Can you work these out from the model? Positions are in its coordinate system, mm. Coordinates: 2 decimals unless noted, no trailing zeros. Order: outer loops, then holes, each group sorted by start corner. A loop starts at its lowest first (then second) coordinate and runs counter-clockwise, first axis right, second up. Notation, with made-up numbers: (71.5, -12) -> (92.5, -12) arc R20 ccw to (92.5, 7) -> close; hole circle Ø7 at (39.5, -17.5). An arc over 180 degrees is marked (long way). Return JSON: item names as keys, results as strings. Group by question number.
1) If we section it at D-D, the plane z = -8: Please give me the cut outline in (x, y).
2) If I drill on probe 1 along Z at (x, y) = (0, 38.6) (3 decimals); probe 2 along Y at (x, z) = (2.25, 0) (3 decimals); probe 3 along Y at (x, z) = (0, -7), over which ranges is the centre line in solid material (lowest first)? Write a range as from..to.
3) If we section it at C-C, the plane x = 0.75: Please give me the cut outline in (y, z) (3 decimals).
4) Thinking about a two-plate mould opening in X: for faces 1 (the flat face through (4, 16, 16)), 2 (the flat face through (-2, 0, 0)), 3 (the cylindrical face through (-0.2, 20.95, -20.86)), 4 (the flat face through (-4, 16, 16)), which applies, +X half, -X half, draft (parallel to the pull), parting line (faces both ways), or undercut?
5) If we section it at A-A, the plane y = 25.5: Please give me the cut outline in (x, z) (1 decimal).
6) If we section it at B-B, the plane z = 0: Please give me the cut outline in (x, y) (1 decimal).
from build123d import *

# Parameters (mm, degrees)
SKETCH2_W           = 8.001
SKETCH2_H           = 45.75
SKETCH2_R           = 1.5
BOSS_EXTRUDE1_DEPTH = 42.5
SKETCH3_R           = 15.875
CUT_EXTRUDE1_DEPTH  = 42.5


with BuildPart() as part:
    # Sketch2 → Boss-Extrude1 (new body)
    with BuildSketch(Plane(origin=(0, 0, 0), x_dir=(1, 0, 0), z_dir=(0, 1, 0))):
        Rectangle(SKETCH2_W, SKETCH2_H)
        Circle(SKETCH2_R, mode=Mode.SUBTRACT)
        with Locations((0, 19.375)):
            Circle(SKETCH2_R, mode=Mode.SUBTRACT)
        with Locations((0, -19.375)):
            Circle(SKETCH2_R, mode=Mode.SUBTRACT)
    extrude(amount=BOSS_EXTRUDE1_DEPTH)

    # Sketch3 → Cut-Extrude1 (cut)
    with BuildSketch(Plane(origin=(4.0005, 0, 0), x_dir=(0, 0, -1), z_dir=(1, 0, 0))):
        with Locations((0, 21.25)):
            Circle(SKETCH3_R)
    extrude(amount=-CUT_EXTRUDE1_DEPTH, mode=Mode.SUBTRACT)


solid = part.part
Result sheet:
{
 "1": {"outline": "(-4, 0) -> (4, 0) -> (4, 7.54) -> (-4, 7.54) -> close; (-4, 34.96) -> (4, 34.96) -> (4, 42.5) -> (-4, 42.5) -> close"},
 "2": {"probe 1": "z = -22.875..-20.875, -17.875..-1.5, 1.5..17.875, 20.875..22.875", "probe 2": "y = 0..5.375, 37.125..42.5", "probe 3": "y = 0..7, 35.5..42.5"},
 "3": {"outline": "(0, -22.875) -> (42.5, -22.875) -> (42.5, -20.674) -> (0, -20.674) -> close; (0, -18.076) -> (42.5, -18.076) -> (42.5, -1.299) -> (37.072, -1.299) arc R15.875 cw to (5.428, -1.299) -> (0, -1.299) -> close; (0, 1.299) -> (5.428, 1.299) arc R15.875 cw to (37.072, 1.299) -> (42.5, 1.299) -> (42.5, 18.076) -> (0, 18.076) -> close; (0, 20.674) -> (42.5, 20.674) -> (42.5, 22.875) -> (0, 22.875) -> close"},
 "4": {"face 1": "+X half", "face 2": "draft", "face 3": "undercut", "face 4": "-X half"},
 "5": {"outline": "(-4, -22.9) -> (4, -22.9) -> (4, -15.3) -> (-4, -15.3) -> close; (-4, 15.3) -> (4, 15.3) -> (4, 22.9) -> (-4, 22.9) -> close; hole circle Ø3 at (0, -19.4); hole circle Ø3 at (0, 19.4)"},
 "6": {"outline": "(-4, 0) -> (-1.5, 0) -> (-1.5, 5.4) -> (-4, 5.4) -> close; (-4, 37.1) -> (-1.5, 37.1) -> (-1.5, 42.5) -> (-4, 42.5) -> close; (1.5, 0) -> (4, 0) -> (4, 5.4) -> (1.5, 5.4) -> close; (1.5, 37.1) -> (4, 37.1) -> (4, 42.5) -> (1.5, 42.5) -> close"}
}
